Input: part model. Units: mm. Frame: model coordinates. Face numbers are marked on the shaded views. Round coordinates to 2 decimals unless told otherwise and drop trailing zeros. Loops run counter-clockwise (first coordinate to the right, second up) from the corner with the lowest first, then second, coordinate; pieces in that order, holes last. Notation, with made-up numbers: M 10,4.5 L 22,4.5 A16 cw 22,9.5 Z; hole C -31.5,74.5 d8. An arc over 180 degrees is marked long. Use one line per item in the form item = value. Start each with the question number.
Q1. Section query B-B, the plane y = 0. Output: boundary loops of the cut face in (x, z), and give its area (3 significant figures).
Q2. Section query A-A, the plane x = 0. Output: boundary loops of the cut face in (y, z), and give its area (3 significant figures).
Q3. First-contact query: P1, Ø5, axis at x = 4, z = 2.5, coming from the +Y side; P2, Ø2, axis at x = -7, z = 2.5, coming from the -Y side. Flat tips, straight axial feed; report the tip coordinate or a pass-through.
Q4. Ray query, line 1 along X through (y, z) = (-39.25, 2.75); line 2 along Y through (x, z) = (13.5, 4.5); line 3 along Y through (x, z) = (-3, 5.5). Return the intervals inside material, ascending.
Q5. Section query C-C, the plane z = 3.25. Output: boundary loops of the cut face in (x, y).
Q6. Section query D-D, the plane x = 14. Output: boundary loops of the cut face in (y, z).
Q7. Mould query, pull axis Y, two halves, no side actions, for the marked faces 1, 2 and 3. Classes: pulls with the +Y half, pulls with the -Y half, needs draft (parallel to the pull), parting line crosses it, or undercut.
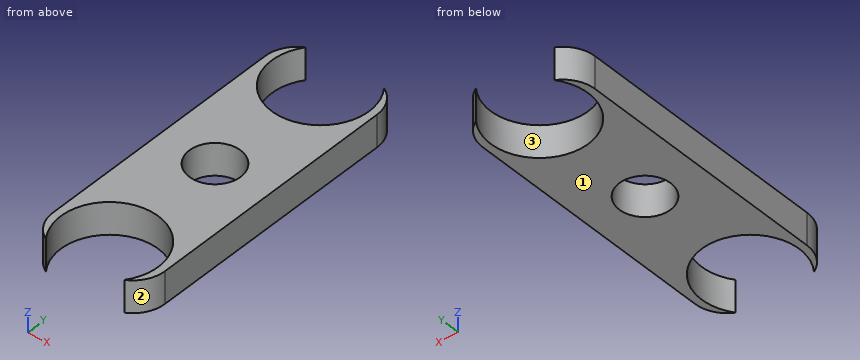
```python
from build123d import *

# Parameters (mm, degrees)
SKETCH1_R           = 8
BOSS_EXTRUDE1_DEPTH = 10
FILLET1_R           = 10


with BuildPart() as part:
    # Sketch1 → Boss-Extrude1 (new body)
    with BuildSketch(Plane(origin=(0, 0, 0), x_dir=(0, 1, 0), z_dir=(0, 0, 1))):
        with BuildLine():
            Line((48.312247408, -17.530203429), (48.312247408, -12.265323963))
            ThreePointArc((48.312247408, -12.265323963), (24, 0), (48.312247408, 12.265323963))
            Line((48.312247408, 12.265323963), (48.312247408, 17.530203429))
            Line((48.312247408, 17.530203429), (-48.312247408, 17.530203429))
            Line((-48.312247408, 17.530203429), (-48.312247408, 12.265323963))
            ThreePointArc((-48.312247408, 12.265323963), (-24, 0), (-48.312247408, -12.265323963))
            Line((-48.312247408, -12.265323963), (-48.312247408, -17.530203429))
            Line((-48.312247408, -17.530203429), (48.312247408, -17.530203429))
        make_face()
        with Locations(Location((0, 0, 0), (0, 0, 270))):
            Circle(SKETCH1_R, mode=Mode.SUBTRACT)
    extrude(amount=BOSS_EXTRUDE1_DEPTH)

    # Fillet1
    # the kernel refuses this fillet: 10 mm, written as the material it takes off along each edge
    with BuildSketch(Plane(origin=(-17.530203429, 48.312247408, -22.019683457), x_dir=(1, 0, 0), z_dir=(0, 0, 1)), Plane(origin=(17.530203429, -48.312247408, -22.019683457), x_dir=(-1, 0, 0), z_dir=(0, 0, 1))) as fillet1_piece_1:
        with BuildLine():
            CenterArc((10, -8.807873383), FILLET1_R, 118.262514111, 61.737485889)
            Line((0, -8.807873383), (-0.2, -8.807873383))
            Line((-0.2, -8.807873383), (-0.2, 0))
            Line((-0.2, 0), (0, 0.2))
            ThreePointArc((0, 0.2), (2.632439733, 0.2), (5.170177055, 0.176157468))
            Line((5.170177055, 0.176157468), (5.264879466, 0))
        make_face()
    extrude(amount=54.039366915, mode=Mode.SUBTRACT)
    with BuildSketch(Plane(origin=(-17.530203429, -48.312247408, -22.019683457), x_dir=(0, 1, 0), z_dir=(0, 0, 1)), Plane(origin=(17.530203429, 48.312247408, -22.019683457), x_dir=(0, -1, 0), z_dir=(0, 0, 1))) as fillet1_piece_2:
        with BuildLine():
            CenterArc((8.807873383, -10), FILLET1_R, 90, 61.737485889)
            Line((0, -5.264879466), (-0.176157468, -5.170177055))
            ThreePointArc((-0.176157468, -5.170177055), (-0.2, -2.632439733), (-0.2, 0))
            Line((-0.2, 0), (0, 0.2))
            Line((0, 0.2), (8.807873383, 0.2))
            Line((8.807873383, 0.2), (8.807873383, 0))
        make_face()
    extrude(amount=54.039366915, mode=Mode.SUBTRACT)


solid = part.part
```
Results found:
q1.outline = M -17.53,0 L -8,0 L -8,10 L -17.53,10 Z; M 8,0 L 17.53,0 L 17.53,10 L 8,10 Z
q1.area = 191 mm²
q2.outline = M -24,0 L -8,0 L -8,10 L -24,10 Z; M 8,0 L 24,0 L 24,10 L 8,10 Z
q2.area = 320 mm²
q3.P1 = 25.45
q3.P2 = -26.27
q4.line_1 = -17.53 to -15.25, 15.25 to 17.53
q4.line_2 = -47.53 to -46.34, -32.16 to 32.16, 46.34 to 47.53
q4.line_3 = -24.3 to -7.42, 7.42 to 24.3
q5.outline = M -17.53,-39.5 A10 ccw -12.27,-48.31 A15.25 cw long 12.27,-48.31 A10 ccw 17.53,-39.5 L 17.53,39.5 A10 ccw 12.27,48.31 A15.25 cw long -12.27,48.31 A10 ccw -17.53,39.5 Z; hole C 0,0 d16
q6.outline = M -47.13,0 L -45.3,0 L -45.3,10 L -47.13,10 Z; M -33.2,0 L 33.2,0 L 33.2,10 L -33.2,10 Z; M 45.3,0 L 47.13,0 L 47.13,10 L 45.3,10 Z
q7.face_1 = needs draft
q7.face_2 = pulls with the -Y half
q7.face_3 = undercut
